```python
from build123d import *

# Parameters (mm, degrees)
F0_W         = 77.9829304665
F0_H         = 47.1442025155
F1_DEPTH     = 50.8
F2_T         = -12.7
F3_T1_DEPTH  = 52.5829304665
F3_T3_DEPTH  = 21.7442025155
F3_T9_DEPTH  = 116.0829304665
F3_T15_DEPTH = 85.2442025155
F3_T24_DEPTH = 116.0829304665
F3_T30_DEPTH = 85.2442025155
F3_T39_DEPTH = 116.0829304665
F3_T45_DEPTH = 85.2442025155
F3_T54_DEPTH = 85.2442025155
F3_T60_DEPTH = 116.0829304665


# Not quite as in the source:
# - a fillet or chamfer that OpenCascade refuses, or shapes differently, is made with other operations: its cross-section is extruded or revolved along the edge and cut away or added


with BuildPart() as f1:
    # F0 (on Top) → F1 (new body)
    with BuildSketch(Plane.XY):
        with Locations((25.9893098846, -0.1163231209)):
            Rectangle(F0_W, F0_H)
    extrude(amount=F1_DEPTH)

    # F2
    f2_openings = [f1.faces().sort_by_distance(p)[0] for p in [
        (25.98931, -0.116323, 50.8),
    ]]
    offset(amount=F2_T, openings=f2_openings)

    # F3: fillet of radius 25.4 on 4 edges, made by hand

    # F3_s2 → F3_t1 (cut)
    with BuildSketch(Plane.YZ.offset(-0.3021553487)):
        with BuildLine():
            ThreePointArc((36.1557781368, 50.8), (18.1952658947, 43.3605122421), (10.7557781368, 25.4))
            Line((10.7557781368, 25.4), (10.7557781368, 50.8))
            Line((10.7557781368, 50.8), (36.1557781368, 50.8))
        make_face()
        with BuildLine():
            ThreePointArc((-36.3884243786, 50.8), (-18.4279121365, 43.3605122421), (-10.9884243786, 25.4))
            Line((-10.9884243786, 25.4), (-10.9884243786, 50.8))
            Line((-10.9884243786, 50.8), (-36.3884243786, 50.8))
        make_face()
    extrude(amount=F3_T1_DEPTH, mode=Mode.SUBTRACT)

    # F3_s4 → F3_t3 (cut)
    with BuildSketch(Plane.XZ.offset(-10.7557781368)):
        with BuildLine():
            ThreePointArc((-25.7021553487, 50.8), (-7.7416431065, 43.3605122421), (-0.3021553487, 25.4))
            Line((-0.3021553487, 25.4), (-0.3021553487, 50.8))
            Line((-0.3021553487, 50.8), (-25.7021553487, 50.8))
        make_face()
        with BuildLine():
            ThreePointArc((77.6807751179, 50.8), (59.7202628757, 43.3605122421), (52.2807751179, 25.4))
            Line((52.2807751179, 25.4), (52.2807751179, 50.8))
            Line((52.2807751179, 50.8), (77.6807751179, 50.8))
        make_face()
    extrude(amount=F3_T3_DEPTH, mode=Mode.SUBTRACT)


with BuildPart() as f3_tool7:
    # F3_s8 → F3_t9 (new body)
    with BuildSketch(Plane.YZ.offset(115.7807751179)):
        with BuildLine():
            ThreePointArc((36.1557781368, 50.8), (18.1952658947, 43.3605122421), (10.7557781368, 25.4))
            Line((10.7557781368, 25.4), (10.7557781368, 50.8))
            Line((10.7557781368, 50.8), (36.1557781368, 50.8))
        make_face()
    extrude(amount=-F3_T9_DEPTH)

    split(bisect_by=Plane.XZ.offset(-23.4557781368), keep=Keep.TOP)

    split(bisect_by=Plane.YZ.offset(64.9807751179), keep=Keep.BOTTOM)

    split(bisect_by=Plane.YZ.offset(52.2807751179), keep=Keep.TOP)


with BuildPart() as f3_tool13:
    # F3_s14 → F3_t15 (new body)
    with BuildSketch(Plane.XZ.offset(10.9884243786)):
        with BuildLine():
            ThreePointArc((77.6807751179, 50.8), (59.7202628757, 43.3605122421), (52.2807751179, 25.4))
            Line((52.2807751179, 25.4), (52.2807751179, 50.8))
            Line((52.2807751179, 50.8), (77.6807751179, 50.8))
        make_face()
    extrude(amount=-F3_T15_DEPTH)

    split(bisect_by=Plane.XZ.offset(-23.4557781368), keep=Keep.TOP)

    split(bisect_by=Plane.YZ.offset(64.9807751179), keep=Keep.BOTTOM)

    split(bisect_by=Plane.XZ.offset(-10.7557781368), keep=Keep.BOTTOM)


with BuildPart() as f3_tool7_1:
    add(f3_tool7.part)

    # F3_t19: intersect F3_tool13
    add(f3_tool13.part, mode=Mode.INTERSECT)


with BuildPart() as f1_1:
    add(f1.part)

    # F3_t5: cut F3_tool7
    add(f3_tool7_1.part, mode=Mode.SUBTRACT)


with BuildPart() as f3_tool22:
    # F3_s23 → F3_t24 (new body)
    with BuildSketch(Plane.YZ.offset(52.2807751179)):
        with BuildLine():
            ThreePointArc((36.1557781368, 50.8), (18.1952658947, 43.3605122421), (10.7557781368, 25.4))
            Line((10.7557781368, 25.4), (10.7557781368, 50.8))
            Line((10.7557781368, 50.8), (36.1557781368, 50.8))
        make_face()
    extrude(amount=-F3_T24_DEPTH)

    split(bisect_by=Plane.XZ.offset(-23.4557781368), keep=Keep.TOP)

    split(bisect_by=Plane.YZ.offset(-13.0021553487), keep=Keep.TOP)

    split(bisect_by=Plane.YZ.offset(-0.3021553487), keep=Keep.BOTTOM)


with BuildPart() as f3_tool28:
    # F3_s29 → F3_t30 (new body)
    with BuildSketch(Plane.XZ.offset(-74.2557781368)):
        with BuildLine():
            ThreePointArc((-25.7021553487, 50.8), (-7.7416431065, 43.3605122421), (-0.3021553487, 25.4))
            Line((-0.3021553487, 25.4), (-0.3021553487, 50.8))
            Line((-0.3021553487, 50.8), (-25.7021553487, 50.8))
        make_face()
    extrude(amount=F3_T30_DEPTH)

    split(bisect_by=Plane.XZ.offset(-23.4557781368), keep=Keep.TOP)

    split(bisect_by=Plane.YZ.offset(-13.0021553487), keep=Keep.TOP)

    split(bisect_by=Plane.XZ.offset(-10.7557781368), keep=Keep.BOTTOM)


with BuildPart() as f3_tool22_1:
    add(f3_tool22.part)

    # F3_t34: intersect F3_tool28
    add(f3_tool28.part, mode=Mode.INTERSECT)


with BuildPart() as f1_2:
    add(f1_1.part)

    # F3_t20: cut F3_tool22
    add(f3_tool22_1.part, mode=Mode.SUBTRACT)


with BuildPart() as f3_tool37:
    # F3_s38 → F3_t39 (new body)
    with BuildSketch(Plane.YZ.offset(-63.8021553487)):
        with BuildLine():
            ThreePointArc((-36.3884243786, 50.8), (-18.4279121365, 43.3605122421), (-10.9884243786, 25.4))
            Line((-10.9884243786, 25.4), (-10.9884243786, 50.8))
            Line((-10.9884243786, 50.8), (-36.3884243786, 50.8))
        make_face()
    extrude(amount=F3_T39_DEPTH)

    split(bisect_by=Plane.YZ.offset(-13.0021553487), keep=Keep.TOP)

    split(bisect_by=Plane.XZ.offset(23.6884243786), keep=Keep.BOTTOM)

    split(bisect_by=Plane.YZ.offset(-0.3021553487), keep=Keep.BOTTOM)


with BuildPart() as f3_tool43:
    # F3_s44 → F3_t45 (new body)
    with BuildSketch(Plane.XZ.offset(-10.7557781368)):
        with BuildLine():
            ThreePointArc((-25.7021553487, 50.8), (-7.7416431065, 43.3605122421), (-0.3021553487, 25.4))
            Line((-0.3021553487, 25.4), (-0.3021553487, 50.8))
            Line((-0.3021553487, 50.8), (-25.7021553487, 50.8))
        make_face()
    extrude(amount=F3_T45_DEPTH)

    split(bisect_by=Plane.YZ.offset(-13.0021553487), keep=Keep.TOP)

    split(bisect_by=Plane.XZ.offset(23.6884243786), keep=Keep.BOTTOM)

    split(bisect_by=Plane.XZ.offset(10.9884243786), keep=Keep.TOP)


with BuildPart() as f3_tool37_1:
    add(f3_tool37.part)

    # F3_t49: intersect F3_tool43
    add(f3_tool43.part, mode=Mode.INTERSECT)


with BuildPart() as f1_3:
    add(f1_2.part)

    # F3_t35: cut F3_tool37
    add(f3_tool37_1.part, mode=Mode.SUBTRACT)


with BuildPart() as f3_tool52:
    # F3_s53 → F3_t54 (new body)
    with BuildSketch(Plane.XZ.offset(74.4884243786)):
        with BuildLine():
            ThreePointArc((77.6807751179, 50.8), (59.7202628757, 43.3605122421), (52.2807751179, 25.4))
            Line((52.2807751179, 25.4), (52.2807751179, 50.8))
            Line((52.2807751179, 50.8), (77.6807751179, 50.8))
        make_face()
    extrude(amount=-F3_T54_DEPTH)

    split(bisect_by=Plane.XZ.offset(23.6884243786), keep=Keep.BOTTOM)

    split(bisect_by=Plane.YZ.offset(64.9807751179), keep=Keep.BOTTOM)

    split(bisect_by=Plane.XZ.offset(10.9884243786), keep=Keep.TOP)


with BuildPart() as f3_tool58:
    # F3_s59 → F3_t60 (new body)
    with BuildSketch(Plane.YZ.offset(-0.3021553487)):
        with BuildLine():
            ThreePointArc((-36.3884243786, 50.8), (-18.4279121365, 43.3605122421), (-10.9884243786, 25.4))
            Line((-10.9884243786, 25.4), (-10.9884243786, 50.8))
            Line((-10.9884243786, 50.8), (-36.3884243786, 50.8))
        make_face()
    extrude(amount=F3_T60_DEPTH)

    split(bisect_by=Plane.XZ.offset(23.6884243786), keep=Keep.BOTTOM)

    split(bisect_by=Plane.YZ.offset(64.9807751179), keep=Keep.BOTTOM)

    split(bisect_by=Plane.YZ.offset(52.2807751179), keep=Keep.TOP)


with BuildPart() as f3_tool52_1:
    add(f3_tool52.part)

    # F3_t64: intersect F3_tool58
    add(f3_tool58.part, mode=Mode.INTERSECT)


with BuildPart() as f1_4:
    add(f1_3.part)

    # F3_t50: cut F3_tool52
    add(f3_tool52_1.part, mode=Mode.SUBTRACT)


solid = f1_4.part
```
Design review of the part built by this model. Coordinates are the model's own, in mm. A direction names the side the tool comes from. Give positions to 0.01 mm unless a question says otherwise; leave off trailing zeros. Order: outer loops, then holes, each group sorted by start corner. A loop starts at its lowest first (then second) coordinate and runs counter-clockwise, first axis right, second up. Notation, with made-up numbers: (2, -10) -> (47, -10) arc R5 ccw to (47, -3) -> close; hole circle Ø8 at (-39, -17.5). An arc over 180 degrees is marked (long way). Write each question's results on one line, items separated by ' | '. Start each with the question number.
Q1. Mouldability with a two-part tool opening along X and no side actions: class faces 1 (the flat face through (64.981, 0, 23)), 2 (the flat face through (52.281, 0, 19)), 3 (the flat face through (-13.002, 0, 23)), 4 (the flat face through (25, 23.456, 23)) as +X half, -X half, draft (parallel to the pull), parting line (faces both ways), or undercut.
Q2. Add section A-A on z = 17.5. Give the boundary of the cut face in (x, y), and give its area (3 significant figures).
Q3. For pin 1 (10 mm diameter, centred on x = 42.5, y = 1, fed in from +Z), flat-tipped, find the tip position at first contact; note if it passes through.
Q4. Machinability: for faces 5 (the flat face through (25, 0, 0)), 6 (the flat face through (-0.302, 0, 19)), which of the approach directions +Z, -Z, +X, -X, +Y, -Y give a long, thin tool a straight path to every point of the face, cutting with its end or side? Answer none if there is none.
Q5. Wall thickness on L1, parallel to Y at x = 33, z = 20; L2, parallel to Z at x = 37, y = -5.5; L3, parallel to X at y = -1.5, z = 15: over which ranges is each line inside the solid? List them lowest first. Write a range as from..to.
Q6. Add section C-C on x = 13. Give the boundary of the cut face in (y, z), and give its area (3 significant figures).
Q7. Add section B-B on y = -6. Give the boundary of the cut face in (x, z), and give its area (3 significant figures).
Q8. Add section D-D on z = 29.5. Give the boundary of the cut face in (x, y).
Found:
1) face 1: +X half | face 2: undercut | face 3: -X half | face 4: draft
2) outline: (-13, -23.69) -> (64.98, -23.69) -> (64.98, 23.46) -> (-13, 23.46) -> close; hole (-0.3, -10.99) -> (52.28, -10.99) -> (52.28, 10.76) -> (-0.3, 10.76) -> close | area: 2,530 mm2
3) pin 1: stops at z = 12.7
4) face 5: -Z, +X, -X, +Y, -Y | face 6: +Z
5) L1: y = -23.69..-10.99, 10.76..23.46 | L2: z = 0..12.7 | L3: x = -13..-0.3, 52.28..64.98
6) outline: (-23.69, 0) -> (23.46, 0) -> (23.46, 47.4) arc R25.4 ccw to (10.76, 25.4) -> (10.76, 12.7) -> (-10.99, 12.7) -> (-10.99, 25.4) arc R25.4 ccw to (-23.69, 47.4) -> close | area: 1,320 mm2
7) outline: (-13, 0) -> (64.98, 0) -> (64.98, 47.4) arc R25.4 ccw to (52.28, 25.4) -> (52.28, 12.7) -> (-0.3, 12.7) -> (-0.3, 25.4) arc R25.4 ccw to (-13, 47.4) -> close | area: 1,710 mm2
8) outline: (-13, -23.69) -> (64.98, -23.69) -> (64.98, 23.46) -> (-13, 23.46) -> close; hole (-0.64, -11.32) -> (52.61, -11.32) -> (52.61, 11.09) -> (-0.64, 11.09) -> close
